from build123d import *

# Parameters (mm, degrees)
SKETCH_1_W          = 60
SKETCH_1_H          = 45
EXTRUDE_1_DEPTH     = 3
SKETCH_2_W          = 60
SKETCH_2_H          = 3
EXTRUDE_2_DEPTH     = 3
SKETCH_3_W          = 20
SKETCH_3_H          = 3
CUT_EXTRUDE_1_DEPTH = 3
EXTRUDE_START       = -39
EXTRUDE_3_DEPTH     = 39
SKETCH_5_R          = 2.5
CUT_EXTRUDE_2_DEPTH = 74.573092908
SKETCH_6_W          = 60
SKETCH_6_H          = 3
CUT_EXTRUDE_3_DEPTH = 74.573092908
SKETCH_8_W          = 20
SKETCH_8_H          = 3
CUT_EXTRUDE_4_DEPTH = 76.325958341
EXTRUDE_4_DEPTH     = 45
EXTRUDE_5_DEPTH     = 45
SKETCH_11_W         = 20
SKETCH_11_H         = 3
CUT_EXTRUDE_5_DEPTH = 3
EXTRUDE_6_DEPTH     = 39
SKETCH_14_R         = 2.5
CUT_EXTRUDE_7_DEPTH = 120.701514193
CUT_EXTRUDE_8_REACH = 122.787
SKETCH_16_R         = 1.55


with BuildPart() as part:
    # 草图1 → 凸台-拉伸1 (new body)
    with BuildSketch(Plane.XY):
        with Locations((30, 22.5)):
            Rectangle(SKETCH_1_W, SKETCH_1_H)
    extrude(amount=EXTRUDE_1_DEPTH)

    # 草图2 → 凸台-拉伸2 (add)
    with BuildSketch(Plane.XY.offset(3)):
        with Locations((30, 40.5)):
            Rectangle(SKETCH_2_W, SKETCH_2_H)
        with Locations((30, 4.5)):
            Rectangle(SKETCH_2_W, SKETCH_2_H)
    extrude(amount=EXTRUDE_2_DEPTH)

    # 草图3 → 切除-拉伸1 (cut)
    with BuildSketch(Plane.XY.offset(3)):
        with Locations((26, 1.5)):
            Rectangle(SKETCH_3_W, SKETCH_3_H)
        with Locations((26, 43.5)):
            Rectangle(SKETCH_3_W, SKETCH_3_H)
    extrude(amount=-CUT_EXTRUDE_1_DEPTH, mode=Mode.SUBTRACT)

    # 草图4 → 凸台-拉伸3 (add)
    with BuildSketch(Plane.XZ.offset(-3).offset(EXTRUDE_START)):
        Polygon((19, 0), (26, -7), (33, 0), align=None)
    extrude(amount=EXTRUDE_3_DEPTH)

    # 草图5 → 切除-拉伸2 (cut, through all)
    with BuildSketch(Plane.XZ.offset(-3)):
        with Locations((26, -1)):
            Circle(SKETCH_5_R)
    extrude(amount=-CUT_EXTRUDE_2_DEPTH, mode=Mode.SUBTRACT)

    # 草图6 → 切除-拉伸3 (cut, through all)
    with BuildSketch(Plane.XZ.offset(-3)):
        with Locations((30, 4.5)):
            Rectangle(SKETCH_6_W, SKETCH_6_H)
    extrude(amount=-CUT_EXTRUDE_3_DEPTH, mode=Mode.SUBTRACT)

    # 草图8 → 切除-拉伸4 (cut, through all)
    with BuildSketch(Plane.XZ):
        with Locations((50, 1.5)):
            Rectangle(SKETCH_8_W, SKETCH_8_H)
    extrude(amount=-CUT_EXTRUDE_4_DEPTH, mode=Mode.SUBTRACT)

    # 草图9 → 凸台-拉伸4 (add, through all)
    with BuildSketch(Plane(origin=(0, 45, 0), x_dir=(1, 0, 0), z_dir=(0, 1, 0))):
        Polygon((40, -3), (92.37, 18.8), (91.217092711, 21.569621776), (38.847092711, -0.230378224), align=None)
    extrude(amount=-EXTRUDE_4_DEPTH)

    # 草图10 → 凸台-拉伸5 (add, through all)
    with BuildSketch(Plane(origin=(0, 45, 0), x_dir=(1, 0, 0), z_dir=(0, 1, 0))):
        with BuildLine():
            Line((92.37, 18.8), (91.217092711, 21.569621776))
            ThreePointArc((91.217092711, 21.569621776), (94.034523676, 21.295868773), (95.37, 18.8))
            Line((95.37, 18.8), (95.37, -45.66))
            Line((95.37, -45.66), (92.37, -45.66))
            Line((92.37, -45.66), (92.37, 18.8))
        make_face()
    extrude(amount=-EXTRUDE_5_DEPTH)

    # 草图11 → 切除-拉伸5 (cut)
    with BuildSketch(Plane(origin=(95.37, 0, 0), x_dir=(0, 0, -1), z_dir=(1, 0, 0))):
        with Locations((-31.16, 1.5)):
            Rectangle(SKETCH_11_W, SKETCH_11_H)
        with Locations((-31.16, 43.5)):
            Rectangle(SKETCH_11_W, SKETCH_11_H)
    extrude(amount=-CUT_EXTRUDE_5_DEPTH, mode=Mode.SUBTRACT)

    # 草图12 → 凸台-拉伸6 (add)
    with BuildSketch(Plane(origin=(0, 42, 0), x_dir=(1, 0, 0), z_dir=(0, 1, 0)).offset(EXTRUDE_START)):
        Polygon((92.37, -21.16), (102.37, -31.16), (92.37, -41.16), align=None)
    extrude(amount=EXTRUDE_6_DEPTH)

    # 草图14 → 切除-拉伸7 (cut, through all)
    with BuildSketch(Plane(origin=(0, 42, 0), x_dir=(1, 0, 0), z_dir=(0, 1, 0))):
        with Locations(Location((96.37, -31.16, 0), (0, 0, 270))):
            Circle(SKETCH_14_R)
    extrude(amount=-CUT_EXTRUDE_7_DEPTH, mode=Mode.SUBTRACT)

    # 草图16 → 切除-拉伸8 (cut, up to next)
    with BuildSketch(Plane(origin=(0, 0, 0), x_dir=(-1, 0, 0), z_dir=(0, 0, -1)), mode=Mode.PRIVATE) as cut_extrude_8_sk1:
        with Locations((-6, 33)):
            Circle(SKETCH_16_R)
    cut_extrude_8_tool1 = extrude(cut_extrude_8_sk1.sketch, amount=-CUT_EXTRUDE_8_REACH, mode=Mode.PRIVATE) & part.part
    # 草图16 → 切除-拉伸8 (cut, up to next)
    with BuildSketch(Plane(origin=(0, 0, 0), x_dir=(-1, 0, 0), z_dir=(0, 0, -1)), mode=Mode.PRIVATE) as cut_extrude_8_sk2:
        with Locations((-6, 12)):
            Circle(SKETCH_16_R)
    cut_extrude_8_tool2 = extrude(cut_extrude_8_sk2.sketch, amount=-CUT_EXTRUDE_8_REACH, mode=Mode.PRIVATE) & part.part
    add(cut_extrude_8_tool1.solids().sort_by_distance((6, 33, 0))[0], mode=Mode.SUBTRACT)
    add(cut_extrude_8_tool2.solids().sort_by_distance((6, 12, 0))[0], mode=Mode.SUBTRACT)


solid = part.part
For this review, take the finished solid that the model builds, in its own axes (mm). A direction names the side the tool comes from. Give positions to 0.01 mm unless a question says otherwise; leave off trailing zeros. Order: outer loops, then holes, each group sorted by start corner. A loop starts at its lowest first (then second) coordinate and runs counter-clockwise, first axis right, second up. Notation, with made-up numbers: M 47.25,69 L 92.25,69 A13 cw 92.25,91 Z; hole C -37.5,20 d6. An arc over 180 degrees is marked long. Answer in a Markdown table with one row per item. Add a question column.
(1) For pin 1 (21.5 mm diameter, centred on y = 28, z = -2.5, fed in from +X); pin 2 (11 mm diameter, centred on x = 95, z = 30, fed in from -Y); pin 3 (8 mm diameter, centred on x = 98, z = 35.5, fed in from +Y), all flat-tipped, find the tip position at first contact; note any pin that passes through.
(2) Consider section D-D on z = 5.5. State the section outline as (x, y) points.
(3) For faces 1 (the face through (95.37, 23, 2)), 2 (the face through (36, 43, 2)), 3 (the face through (16, 1, 2)), 4 (the face through (20, 23, 3)), 5 (the face through (65.672, 22.815, -10.936)), list the 3-axis set-ups (+Z, -Z, +X, -X, +Y, -Y) from which the entire face can be reached by the end or side of a thin tool; tool diameter is ignored.
(4) Consider section B-B on x = 6. State the section outline as (y, z) points.
(5) Consider section C-C on y = 25. State the section outline as (x, z) points, and give its area (3 significant figures).
(6) Consider section A-A on y = 33. State the section outline as (x, z) points, and give its area (3 significant figures).
(7) Mouldability with a two-part tool opening along Z and no side actions: class faces 6 (the face through (92.37, 23, 14)), 7 (the face through (94, 43, 21.16)), 8 (the face through (29, 23, -4)) as +Z half, -Z half, draft (parallel to the pull), parting line (faces both ways), or undercut.
(8) Wall thickness on probe 1 along Z at (x, y) = (26, 23); probe 2 along Y at (x, z) = (6, 2.3); probe 3 along X at (y, z) = (23, 31.16): over which ranges is each line inside the solid? List them lowest first. Write a range as [from, to].
Evaluation:
| question | item | result |
|---|---|---|
| 1 | pin 1 | stops at x = 95.37 |
| 1 | pin 2 | stops at y = 3 |
| 1 | pin 3 | stops at y = 42 |
| 2 | outline | M 92.37,0 L 95.37,0 L 95.37,45 L 92.37,45 Z |
| 3 | face 1 | -Z, +X, +Y, -Y |
| 3 | face 2 | +Z, -Z, +Y |
| 3 | face 3 | +Z, -Z, -Y |
| 3 | face 4 | +Z, -X, +Y, -Y |
| 3 | face 5 | -Z, +Y, -Y |
| 4 | outline | M 0,0 L 10.45,0 L 10.45,3 L 0,3 Z; M 13.55,0 L 31.45,0 L 31.45,3 L 13.55,3 Z; M 34.55,0 L 45,0 L 45,3 L 34.55,3 Z |
| 5 | outline | M 0,0 L 19,0 L 26,-7 L 33,0 L 39.4,0 L 91.22,-21.57 A3 ccw 95.37,-18.8 L 95.37,24.16 L 102.37,31.16 L 95.37,38.16 L 95.37,45.66 L 92.37,45.66 L 92.37,-18.8 L 40,3 L 0,3 Z; hole C 26,-1 d5; hole C 96.37,31.16 d5 |
| 5 | area | 549 mm^2 |
| 6 | outline | M 0,0 L 4.45,0 L 4.45,3 L 0,3 Z; M 7.55,0 L 19,0 L 26,-7 L 33,0 L 39.4,0 L 91.22,-21.57 A3 ccw 95.37,-18.8 L 95.37,24.16 L 102.37,31.16 L 95.37,38.16 L 95.37,45.66 L 92.37,45.66 L 92.37,-18.8 L 40,3 L 7.55,3 Z; hole C 26,-1 d5; hole C 96.37,31.16 d5 |
| 6 | area | 540 mm^2 |
| 7 | face 6 | draft |
| 7 | face 7 | undercut |
| 7 | face 8 | -Z half |
| 8 | probe 1 | z = [-7, -3.5], [1.5, 3] |
| 8 | probe 2 | y = [0, 10.45], [13.55, 31.45], [34.55, 45] |
| 8 | probe 3 | x = [92.37, 93.87], [98.87, 102.37] |
